Read the model definition and answer for the solid it produces. Units are mm, in the model's axes. Face numbers are marked on the shaded views. A direction names the side the tool comes from. Round coordinates to 2 decimals unless told otherwise and drop trailing zeros. Loops run counter-clockwise (first coordinate to the right, second up) from the corner with the lowest first, then second, coordinate; pieces in that order, holes last. Notation, with made-up numbers: (-7, 26) -> (24, 26) arc R14 cw to (24, 30) -> close; hole circle Ø3 at (15.5, -34.75). An arc over 180 degrees is marked (long way). Put each result on its own line as item: value.
from build123d import *

# Parameters (mm, degrees)
F0_R     = 2.75
F1_DEPTH = 7
F2_R     = 2.75
F2_R_2   = 2.5
F3_DEPTH = 6
F4_R     = 2.75
F4_R_2   = 2.5
F5_DEPTH = 6


with BuildPart() as f1:
    # F0 (on Front) → F1 (new body, symmetric)
    with BuildSketch(Plane.XZ):
        Circle(F0_R)
    extrude(amount=F1_DEPTH, both=True)

    # F2 (on face) → F3 (cut)
    with BuildSketch(Plane.XZ.offset(7)):
        Circle(F2_R)
        Circle(F2_R_2, mode=Mode.SUBTRACT)
    extrude(amount=-F3_DEPTH, mode=Mode.SUBTRACT)

    # F4 (on face) → F5 (cut)
    with BuildSketch(Plane(origin=(0, 7, 0), x_dir=(-1, 0, 0), z_dir=(0, 1, 0))):
        Circle(F4_R)
        Circle(F4_R_2, mode=Mode.SUBTRACT)
    extrude(amount=-F5_DEPTH, mode=Mode.SUBTRACT)


solid = f1.part
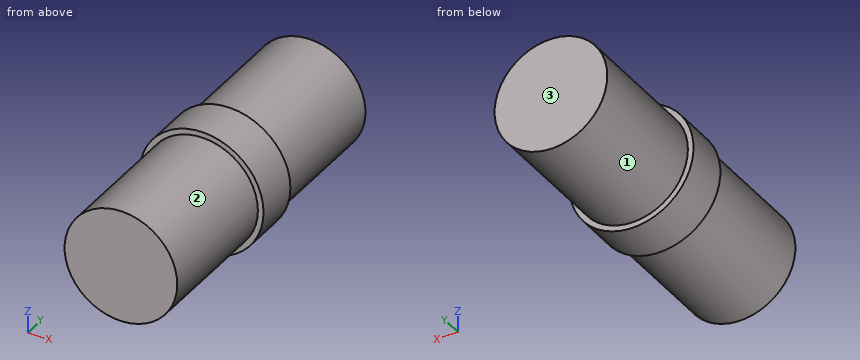
Item 1: The part is cut by section B-B (z = 0). Determine the outline of the cut face in (x, y).
Derived:
outline: (-2.75, -1) -> (-2.5, -1) -> (-2.5, -7) -> (2.5, -7) -> (2.5, -1) -> (2.75, -1) -> (2.75, 1) -> (2.5, 1) -> (2.5, 7) -> (-2.5, 7) -> (-2.5, 1) -> (-2.75, 1) -> close
Item 2: The part is cut by section D-D (y = -3.5). Determine the outline of the cut face in (x, z), then the cut area to 3 significant figures.
Derived:
outline: circle Ø5 at (0, 0)
area: 19.6 mm^2
Item 3: The part is cut by section A-A (x = 0). Determine the outline of the cut face in (y, z), then the cut area to 3 significant figures.
Derived:
outline: (-7, -2.5) -> (-1, -2.5) -> (-1, -2.75) -> (1, -2.75) -> (1, -2.5) -> (7, -2.5) -> (7, 2.5) -> (1, 2.5) -> (1, 2.75) -> (-1, 2.75) -> (-1, 2.5) -> (-7, 2.5) -> close
area: 71.0 mm^2
Item 4: Which of the six approach directions +Z, -Z, +X, -X, +Y, -Y give full straight-line access (tool end or side, diameter ignored) to the marked faces 1, 2 and 3?
Derived:
face 1: +Y
face 2: -Y
face 3: +Z, -Z, +X, -X, +Y
Item 5: Flat-ended cylindrical pins translate along their axes: pin 1 Ø1 at (y, z) = (4, 2) entering from +X; pin 2 Ø1.5 at (x, y) = (-0.5, -3) entering from +Z; pin 3 Ø3 at (x, y) = (-1.5, -0.5) entering from +Z; pin 4 Ø3 at (y, z) = (5, -0.5) entering from +X. Find the tip coordinate at first contact, or state that the pin passes through.
Derived:
pin 1: stops at x = 2
pin 2: stops at z = 2.5
pin 3: stops at z = 2.75
pin 4: stops at x = 2.5
Item 6: Find the intervals of material crossed by line 1 along Y through (x, z) = (0.95, -2.35); line 2 along X through (y, z) = (5.25, -0.1), in increasing order.
Derived:
line 1: y = -1 to 1
line 2: x = -2.5 to 2.5
Item 7: The part is cut by section C-C (y = -0.25). Determine the outline of the cut face in (x, z), then the cut area to 3 significant figures.
Derived:
outline: circle Ø5.5 at (0, 0)
area: 23.8 mm^2
